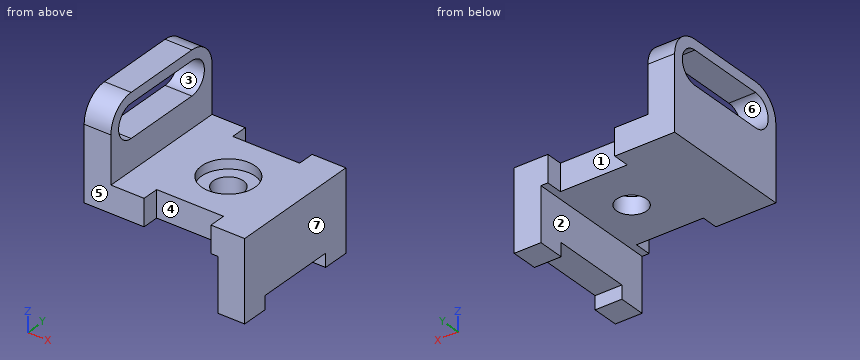
```python
from build123d import *

# Parameters (mm, degrees)
F0_R     = 7.112
F1_DEPTH = 12.7
F3_DEPTH = 12.7
F4_R     = 12.7
F5_DEPTH = 4.572
F7_DEPTH = 12.7


with BuildPart() as f1:
    # F0 (on Top) → F1 (new body)
    with BuildSketch(Plane.XY):
        Polygon((0, 63.5), (0, 0), (15.748, 0), (15.748, 7.874), (47.498, 7.874), (47.498, 0), (63.5, 0), (63.5, 63.5), (47.498, 63.5), (47.498, 55.626), (15.748, 55.626), (15.748, 63.5), align=None)
        with Locations((31.75, 31.75)):
            Circle(F0_R, mode=Mode.SUBTRACT)
    extrude(amount=F1_DEPTH)

    # F2 (on face) → F3 (join)
    with BuildSketch(Plane.YZ.offset(63.5)):
        Polygon((0, -19.05), (0, -25.4), (12.7, -25.4), (12.7, -19.05), (50.8, -19.05), (50.8, -25.4), (63.5, -25.4), (63.5, -19.05), (63.5, 0), (0, 0), align=None)
    extrude(amount=-F3_DEPTH)

    # F4 (on face) → F5 (cut)
    with BuildSketch(Plane.XY.offset(12.7)):
        with Locations((31.75, 31.75)):
            Circle(F4_R)
    extrude(amount=-F5_DEPTH, mode=Mode.SUBTRACT)

    # F6 (on face) → F7 (join)
    with BuildSketch(Plane(origin=(0, 0, 0), x_dir=(0, -1, 0), z_dir=(-1, 0, 0))):
        with BuildLine():
            Line((-63.5, 0), (0, 0))
            Line((0, 0), (0, 35.052))
            ThreePointArc((0, 35.052), (-3.719744, 44.032256), (-12.7, 47.752))
            Line((-12.7, 47.752), (-50.8, 47.752))
            ThreePointArc((-50.8, 47.752), (-59.780256, 44.032256), (-63.5, 35.052))
            Line((-63.5, 35.052), (-63.5, 0))
        make_face()
        with BuildLine():
            ThreePointArc((-50.8, 27.178), (-58.674, 35.052), (-50.8, 42.926))
            Line((-50.8, 42.926), (-12.7, 42.926))
            ThreePointArc((-12.7, 42.926), (-4.826, 35.052), (-12.7, 27.178))
            Line((-12.7, 27.178), (-50.8, 27.178))
        make_face(mode=Mode.SUBTRACT)
    extrude(amount=F7_DEPTH)


solid = f1.part
```
Could you check a few things on this model? Use its own coordinates, in mm. Face numbers are marked on the shaded views. A direction names the side the tool comes from. Give positions to 0.01 mm unless a question says otherwise; leave off trailing zeros. Loops run counter-clockwise (first coordinate to the right, second up) from the corner with the lowest first, then second, coordinate; pieces in that order, holes last. Notation, with made-up numbers: (57.5, 38.5) - (68.5, 38.5) arc R14 cw to (68.5, 54.5) - close; hole circle Ø5 at (71, 88). An arc over 180 degrees is marked (long way). Use one line per item in the form item = value.
1. I'm going to push flat-ended pins straight in: pin 1 Ø12 at (x, y) = (4, 29.5) entering from +Z; pin 2 Ø19 at (x, y) = (4.5, 44) entering from -Z; pin 3 Ø8.5 at (x, y) = (31.75, 31.75) entering from -Z; pin 4 Ø4 at (x, z) = (32.5, 3.5) entering from -Y. Where does each tip first touch, or does it pass through?
Response values:
pin_1 = 47.75
pin_2 = 0
pin_3 = through
pin_4 = 7.87
2. I want a section at B-B (x = 31.75). Please give me the cut outline in (y, z).
Response values:
outline = (7.87, 0) - (24.64, 0) - (24.64, 8.13) - (19.05, 8.13) - (19.05, 12.7) - (7.87, 12.7) - close; (38.86, 0) - (55.63, 0) - (55.63, 12.7) - (44.45, 12.7) - (44.45, 8.13) - (38.86, 8.13) - close
3. I want a section at D-D (z = 17.5). Please give me the cut outline in (x, y).
Response values:
outline = (-12.7, 0) - (0, 0) - (0, 63.5) - (-12.7, 63.5) - close
4. On a 3-axis mill with a long thin cutter (end or side, diameter ignored), from which of +Z, -Z, +X, -X, +Y, -Y can I reach the whole of each face in a straight line? I mean the marked faces 1, 2, 3 and 4. Say none if no direction works.
Response values:
face_1 = +Z, -Z, +Y
face_2 = -Z, -X, +Y, -Y
face_3 = +X, -X
face_4 = +Z, -Z, -Y
5. I want a section at C-C (y = 40). Please give me the cut outline in (x, z).
Response values:
outline = (-12.7, 0) - (50.8, 0) - (50.8, -19.05) - (63.5, -19.05) - (63.5, 12.7) - (41.41, 12.7) - (41.41, 8.13) - (22.09, 8.13) - (22.09, 12.7) - (0, 12.7) - (0, 27.18) - (-12.7, 27.18) - close; (-12.7, 42.93) - (0, 42.93) - (0, 47.75) - (-12.7, 47.75) - close
6. I want a section at A-A (y = 31.75). Please give me the cut outline in (x, z).
Response values:
outline = (-12.7, 0) - (24.64, 0) - (24.64, 8.13) - (19.05, 8.13) - (19.05, 12.7) - (0, 12.7) - (0, 27.18) - (-12.7, 27.18) - close; (-12.7, 42.93) - (0, 42.93) - (0, 47.75) - (-12.7, 47.75) - close; (38.86, 0) - (50.8, 0) - (50.8, -19.05) - (63.5, -19.05) - (63.5, 12.7) - (44.45, 12.7) - (44.45, 8.13) - (38.86, 8.13) - close
7. I need wall thicknesses on probe 1 along X at (y, z) = (31.75, 4.75); probe 2 along Z at (x, y) = (3.5, 53.5); probe 3 along Z at (x, y) = (53, 55). Which ranges of each line are inside material? Lowest first, please.
Response values:
probe_1 = -12.7 to 24.64, 38.86 to 63.5
probe_2 = 0 to 12.7
probe_3 = -25.4 to 12.7
8. Thinking about a two-plate mould opening in Y: for the marked faces 5, 6 and 7, which applies, released by +Y, released by -Y, zero draft, split by the parting line, or undercut?
Response values:
face_5 = released by -Y
face_6 = undercut
face_7 = zero draft
